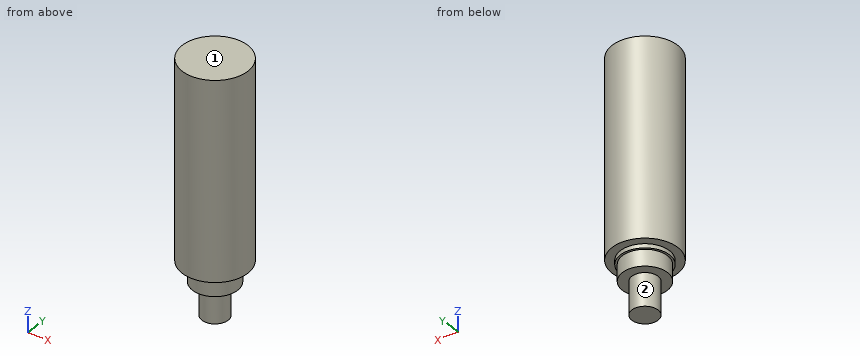
from build123d import *

# Parameters (mm, degrees)
BODYSKE_R    = 4
BODY_DEPTH   = 24
PADSKE_R     = 3
PAD_DEPTH    = 0.5
THREADSKE_R  = 2.75
THREAD_DEPTH = 2
AXISSKE_R    = 1.6
AXIS_DEPTH   = 4


with BuildPart() as part:
    # BodySke → Body (new body)
    with BuildSketch(Plane.XY):
        Circle(BODYSKE_R)
    extrude(amount=BODY_DEPTH)

    # PadSke → Pad (add)
    with BuildSketch(Plane(origin=(0, 0, 0), x_dir=(-1, 0, 0), z_dir=(0, 0, -1))):
        Circle(PADSKE_R)
    extrude(amount=PAD_DEPTH)

    # ThreadSke → Thread (add)
    with BuildSketch(Plane(origin=(0, 0, -0.5), x_dir=(-1, 0, 0), z_dir=(0, 0, -1))):
        Circle(THREADSKE_R)
    extrude(amount=THREAD_DEPTH)

    # AxisSke → Axis (add)
    with BuildSketch(Plane(origin=(0, 0, -2.5), x_dir=(-1, 0, 0), z_dir=(0, 0, -1))):
        Circle(AXISSKE_R)
    extrude(amount=AXIS_DEPTH)


solid = part.part
Verification items for the finished model (mm, model axes). Face numbers are marked on the shaded views. A direction names the side the tool comes from. Coordinates: 2 decimals unless noted, no trailing zeros. Loops run counter-clockwise (first coordinate to the right, second up) from the corner with the lowest first, then second, coordinate; pieces in that order, holes last. Notation, with made-up numbers: (74.5, -31) -> (107.5, -31) arc R17 ccw to (107.5, 1) -> close; hole circle Ø4 at (63.5, 38). An arc over 180 degrees is marked (long way). Answer as a JSON object with one key per item and string values. Group by question number.
Item 1: Tool access check on the marked faces 1 and 2. Record the directions out of +Z, -Z, +X, -X, +Y, -Y that give a thin tool (end or side, any length) a straight path to the whole face; none if there is none.
Item 2: Sectioned sample at C-C on z = 13.5. Record the boundary of the cut face in (x, y), plus the area to 3 significant figures.
Item 3: Scan lines: probe 1 along Z at (x, y) = (-3, 1.5); probe 2 along Z at (x, y) = (1, -2.25); probe 3 along X at (y, z) = (-0.25, 15.5). Record each from-to range of solid material in increasing order.
Item 4: Sectioned sample at A-A on y = 0. Record the boundary of the cut face in (x, z).
Item 5: Depth check by flat-ended pin: pin 1 (4 mm diameter, centred on x = 1.5, z = 12, fed in from +Y); pin 2 (4 mm diameter, centred on x = 2.5, z = 15.5, fed in from -Y). Enter the tip coordinate at first touch or a pass-through.
Evaluation:
{
 "1": {"face 1": "+Z, +X, -X, +Y, -Y", "face 2": "-Z"},
 "2": {"outline": "circle Ø8 at (0, 0)", "area": "50.3 mm²"},
 "3": {"probe 1": "z = 0 to 24", "probe 2": "z = -2.5 to 24", "probe 3": "x = -3.99 to 3.99"},
 "4": {"outline": "(-4, 0) -> (-3, 0) -> (-3, -0.5) -> (-2.75, -0.5) -> (-2.75, -2.5) -> (-1.6, -2.5) -> (-1.6, -6.5) -> (1.6, -6.5) -> (1.6, -2.5) -> (2.75, -2.5) -> (2.75, -0.5) -> (3, -0.5) -> (3, 0) -> (4, 0) -> (4, 24) -> (-4, 24) -> close"},
 "5": {"pin 1": "stops at y = 4", "pin 2": "stops at y = -3.97"}
}
